Can you work these out from the model? Positions are in its coordinate system, mm. A direction names the side the tool comes from. Round coordinates to 2 decimals unless told otherwise and drop trailing zeros. Write each loop counter-clockwise with the first axis right and the second up, starting at its lowest first coordinate (ties: lowest second). Pieces come first, ordered by that corner, then holes. Notation, with made-up numbers: M -32.75,-35 L -23.75,-35 A14 cw -23.75,-31 Z; hole C 54.25,16 d2. An arc over 180 degrees is marked long. Use one line per item in the form item = value. Start each with the question number.
```python
from build123d import *


with BuildPart() as part:
    # Sketch1 → Revolve1 (revolve)
    with BuildSketch(Plane.XY):
        with BuildLine():
            Line((-32.130708731, -1), (-34, 0))
            ThreePointArc((-34, 0), (-35, -1), (-34, -2))
            Line((-34, -2), (-32, -14))
            Line((-32, -14), (-20, -77))
            Line((-20, -77), (-12.6, -77))
            Line((-12.6, -77), (-12.322608601, -76.778086881))
            ThreePointArc((-12.322608601, -76.778086881), (-12.290715274, -76.666899306), (-12.385078106, -76.6))
            Line((-12.385078106, -76.6), (-12.6, -76.6))
            Line((-12.6, -76.6), (-12.6, -75.2))
            Line((-12.6, -75.2), (0, -75.2))
            Line((0, -75.2), (0, -73.7))
            Line((0, -73.7), (-18.592613493, -73.7))
            Line((-18.592613493, -73.7), (-29.964042064, -14))
            Line((-29.964042064, -14), (-32.130708731, -1))
        make_face()
    revolve(axis=Axis((0, 0, 0), (0, -1, 0)))


solid = part.part
```
1. Which directions (+Z, -Z, +X, -X, +Y, -Y) give clear straight access to the entire face, cutting with the end or side of a thin tool? Please do faces 1 (the face through (-28.94, -11.74, -9.11)), 2 (the face through (9.999, -75.89, 7.667)).
2. If we section it at C-C (y = -45.5): List the corners of the cut face in (x, z) for me, and give its area (3 significant figures).
3. If we section it at A-A (z = 0): List the corners of the cut face in (x, y) for me, and give its area (3 significant figures).
4. If we mould it in two halves opening along Z, with no side actions, what happens to faces 3 (the face through (0, -75.2, 0)), 4 (the face through (-30.615, -13.417, -9.641)), 5 (the face through (0, -73.7, 0)), 6 (the face through (-13, -77, 0))? For each: pulls with the +Z half, pulls with the -Z half, needs draft (parallel to the pull), parting line crosses it, or undercut.
5. Please list where these lines run through material, in increasing order: line 1 along Z through (x, y) = (1, -14); line 2 along Y through (x, z) = (7, -11.5); line 3 along Z through (x, y) = (-18.5, -25).
6. If we section it at D-D (y = -6.5): List the corners of the cut face in (x, z) for me.
7. If we section it at B-B (x = 0): List the corners of the cut face in (y, z) for me.
8. Will these pins go through, and if not, where does the flat tip stop? pin 1 (6 mm diameter, centred on x = -14, y = -47.5, fed in from -Z); pin 2 (10 mm diameter, centred on x = -12, y = -59, fed in from -Z); pin 3 (3 mm diameter, centred on x = 7, y = -8, fed in from +Z).
Model answer:
q1.face_1 = +Y
q1.face_2 = none
q2.outline = C 0,0 d52; hole C 0,0 d47.93
q2.area = 320 mm2
q3.outline = M -34,-2 L -32,-14 L -20,-77 L -12.6,-77 L -12.32,-76.78 A0.1 ccw -12.39,-76.6 L -12.6,-76.6 L -12.6,-75.2 L 12.6,-75.2 L 12.6,-76.6 L 12.39,-76.6 A0.1 ccw 12.32,-76.78 L 12.6,-77 L 20,-77 L 32,-14 L 34,-2 A1 ccw 34,0 L 32.13,-1 L 29.96,-14 L 18.59,-73.7 L -18.59,-73.7 L -29.96,-14 L -32.13,-1 L -34,0 A1 ccw Z
q3.area = 390 mm2
q4.face_3 = undercut
q4.face_4 = parting line crosses it
q4.face_5 = undercut
q4.face_6 = needs draft
q5.line_1 = -31.98 to -29.95, 29.95 to 31.98
q5.line_2 = -77 to -73.7
q5.line_3 = -23.5 to -20.84, 20.84 to 23.5
q6.outline = C 0,0 d66.5; hole C 0,0 d62.43
q7.outline = M -77,-20 L -14,-32 L -2,-34 A1 ccw 0,-34 L -1,-32.13 L -14,-29.96 L -73.7,-18.59 L -73.7,18.59 L -14,29.96 L -1,32.13 L 0,34 A1 ccw -2,34 L -14,32 L -77,20 L -77,12.6 L -76.78,12.32 A0.1 ccw -76.6,12.39 L -76.6,12.6 L -75.2,12.6 L -75.2,-12.6 L -76.6,-12.6 L -76.6,-12.39 A0.1 ccw -76.78,-12.32 L -77,-12.6 Z
q8.pin_1 = -23.27
q8.pin_2 = -22.64
q8.pin_3 = 32.64
